Autodesk Inventor part; units mm, degrees
ref_plane "A4_XY" through (220, 0, 0) normal (0, 1, 0) x (1, 0, 0)
ref_plane "A4_YZ" through (220, 0, 0) normal (1, 0, 0) x (0, 0, -1)
ref_plane "A4_ZX" through (220, 0, 0) normal (0, 0, -1) x (0, 1, 0)
sketch "Sketch_1" plane through (0, 0, 0) normal (0, 0, 1) x (1, 0, 0)
  line L0 (92, 0) -> (-48, 0)
  line L1 (-48, 0) -> (-48, 4.233)
  line L2 (-48, 4.233) -> (-47.233, 5)
  line L3 (-47.233, 5) -> (-28.767, 5)
  line L4 (-28.767, 5) -> (-28, 4.233)
  line L5 (-28, 4.233) -> (-28, 4.2)
  line L6 (-28, 4.2) -> (-26, 4.2)
  line L7 (-26, 4.2) -> (-26, 5)
  line L8 (-26, 5) -> (-24.2679, 6)
  line L9 (-24.2679, 6) -> (82, 6)
  line L10 (82, 6) -> (82, 16)
  line L11 (82, 16) -> (92, 16)
  line L12 (92, 16) -> (92, 0)
  line L13 (92, 0) -> (-48, 0)
revolve "Revolution1" add sketch "Sketch_1" angle 360 about axis through (92, 0, 0) along (1, 0, 0)
thread "Thread1"
sketch "Sketch_4" plane through (-26, 0, 0) normal (1, 0, 0) x (0, 0, -1)
  line L0 (-13, -10) -> (13, -10)
  line L1 (13, -10) -> (13, 10)
  line L2 (13, 10) -> (-13, 10)
  line L3 (-13, 10) -> (-13, -10)
  line L4 (-8, 5) -> (-8, -5)
  line L5 (-8, -5) -> (8, -5)
  line L6 (8, -5) -> (8, 5)
  line L7 (8, 5) -> (-8, 5)
extrude "Extrusion1" cut sketch "Sketch_4" along normal blind 6
ref_plane "A4_XY" through (220, 0, 0) normal (0, 1, 0) x (1, 0, 0)
ref_plane "A4_YZ" through (220, 0, 0) normal (1, 0, 0) x (0, 0, -1)
ref_plane "A4_ZX" through (220, 0, 0) normal (0, 0, -1) x (0, 1, 0)
ref_plane "ROD_BODY_XY" through (0, 0, 0) normal (1, 0, 0) x (0, 0, -1)
ref_plane "ROD_BODY_YZ" through (0, 0, 0) normal (0, 0, -1) x (0, 1, 0)
ref_plane "ROD_BODY_ZX" through (0, 0, 0) normal (0, 1, 0) x (1, 0, 0)
ref_plane "ROD_NUT_XY" through (-48, 0, 0) normal (-1, 0, 0) x (0, 0, -1)
ref_plane "ROD_NUT_YZ" through (-48, 0, 0) normal (0, 0, -1) x (0, -1, 0)
ref_plane "ROD_NUT_ZX" through (-48, 0, 0) normal (0, -1, 0) x (-1, 0, 0)
properties part number "CP96S32-50_ROD"
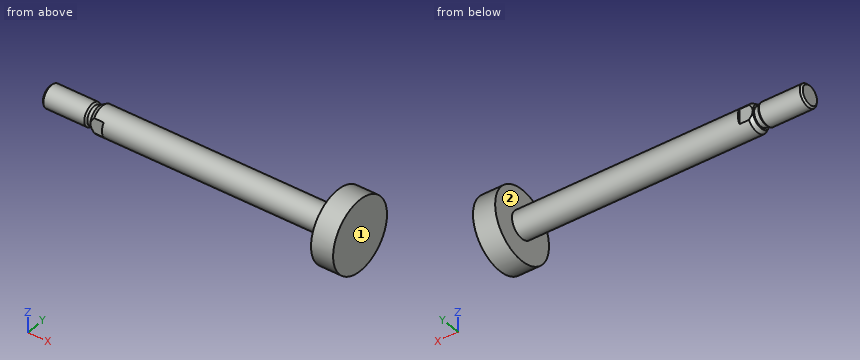
Read the model definition and answer for the solid it produces. Units are mm, in the model's axes. Face numbers are marked on the shaded views. A direction names the side the tool comes from. Give positions to 0.01 mm unless a question says otherwise; leave off trailing zeros. Write each loop counter-clockwise with the first axis right and the second up, starting at its lowest first coordinate (ties: lowest second). Pieces come first, ordered by that corner, then holes. Notation, with made-up numbers: (6.5, 15.5) -> (16.5, 15.5) arc R25 ccw to (16.5, 49.5) -> close; hole circle Ø7 at (77, -21). An arc over 180 degrees is marked (long way). Answer as a JSON object with one key per item and string values.
1) Flat-ended cylindrical pins translate along their axes: pin 1 Ø3 at (x, z) = (7.5, 6.5) entering from +Y; pin 2 Ø1 at (x, z) = (49, -1.5) entering from -Y; pin 3 Ø6 at (x, y) = (37, -11.5) entering from -Z; pin 4 Ø3 at (x, z) = (-23, -1) entering from -Y. Find the tip coordinate at first contact, or state that the pin passes through.
Findings below:
{"pin 1": "stops at y = 3.32", "pin 2": "stops at y = -5.92", "pin 3": "passes through", "pin 4": "stops at y = -5"}
2) Section D-D on x = 66.5 is taken. Write down the section's boundary in (y, z), then the cut area to 3 significant figures.
Findings below:
{"outline": "circle Ø12 at (0, 0)", "area": "113 mm^2"}
3) A tool of negligible diameter and unlimited length cuts with its end or side. For the marked faces 1 and 2, from which of +Z, -Z, +X, -X, +Y, -Y can it reach the whole face along a straight path? Write none if from no direction.
Findings below:
{"face 1": "+Z, -Z, +X, +Y, -Y", "face 2": "-X"}
4) Section C-C on z = 12 is taken. Write down the section's boundary in (x, y).
Findings below:
{"outline": "(82, -10.58) -> (92, -10.58) -> (92, 10.58) -> (82, 10.58) -> close"}
5) Section B-B on x = -31.5 is taken. Write down the section's boundary in (y, z), then the cut area to 3 significant figures.
Findings below:
{"outline": "circle Ø10 at (0, 0)", "area": "78.5 mm^2"}
6) Straight lines are drawn through the part: probe 1 along X at (y, z) = (-9.5, -2); probe 2 along Z at (x, y) = (70.5, -5). For each, find the intervals that lie inside material, in ascending order. Write a range as from..to.
Findings below:
{"probe 1": "x = 82..92", "probe 2": "z = -3.32..3.32"}
